from build123d import *

# Parameters (mm, degrees)
F1_DEPTH = 38.1


# Not quite as in the source:
# - the program builds the solid bodies; features that only make, move or delete a surface that nothing else refers to are left out


with BuildPart() as f1:
    # F0 (on Front) → F1 (new body)
    with BuildSketch(Plane.XZ):
        with BuildLine():
            Line((-12.4957701793, -2.2684196318), (12.4957701793, -2.2684196318))
            ThreePointArc((12.4957701793, -2.2684196318), (0, 12.7), (-12.4957701793, -2.2684196318))
        make_face()
        with BuildLine():
            Line((12.4957701793, -7.3484196318), (12.4957701793, -2.2684196318))
            Line((12.4957701793, -2.2684196318), (-12.4957701793, -2.2684196318))
            Line((-12.4957701793, -2.2684196318), (-49.8945600124, -2.2684196318))
            ThreePointArc((-49.8945600124, -2.2684196318), (-50.3994056233, -4.9895144213), (-51.8467453044, -7.3484196318))
            Line((-51.8467453044, -7.3484196318), (12.4957701793, -7.3484196318))
        make_face()
        with BuildLine():
            ThreePointArc((-51.8467453044, -7.3484196318), (-50.3994056233, -4.9895144213), (-49.8945600124, -2.2684196318))
            Line((-49.8945600124, -2.2684196318), (-57.4802711475, -2.2684196318))
            Line((-57.4802711475, -2.2684196318), (-57.4802711475, -7.3484196318))
            Line((-57.4802711475, -7.3484196318), (-51.8467453044, -7.3484196318))
        make_face()
        with BuildLine():
            Line((-57.4802711475, -2.2684196318), (-49.8945600124, -2.2684196318))
            ThreePointArc((-49.8945600124, -2.2684196318), (-64.5611366718, 0.4526751578), (-51.8467453044, -7.3484196318))
            Line((-51.8467453044, -7.3484196318), (-57.4802711475, -7.3484196318))
            Line((-57.4802711475, -7.3484196318), (-57.4802711475, -2.2684196318))
        make_face()
    extrude(amount=F1_DEPTH)


solid = f1.part
Work out the finished part from the listing and answer in its coordinate system (mm). A direction names the side the tool comes from. Coordinates: 2 decimals unless noted, no trailing zeros. Loops run counter-clockwise (first coordinate to the right, second up) from the corner with the lowest first, then second, coordinate; pieces in that order, holes last. Notation, with made-up numbers: (14, 44) -> (35, 44) arc R20 ccw to (35, 49) -> close; hole circle Ø3 at (36.25, 69). An arc over 180 degrees is marked (long way). Answer as CSV lines item,"result".
1) Straight lines are drawn through the part: probe 1 along Z at (x, y) = (-46, -11); probe 2 along X at (y, z) = (-21, -1.5); probe 3 along X at (y, z) = (-8.5, 2.75). For each, find the intervals that lie inside material, in ascending order.
A:
probe 1,"z = -7.35 to -2.27"
probe 2,"x = -65.03 to -49.93, -12.61 to 12.61"
probe 3,"x = -63.17 to -51.79, -12.4 to 12.4"
2) Flat-ended cylindrical pins translate along their axes: pin 1 (3 mm diameter, centred on x = -54, y = -19, fed in from -Z); pin 2 (11.5 mm diameter, centred on x = -35.5, y = -12, fed in from -Z); pin 3 (18.5 mm diameter, centred on x = -27, y = -19.5, fed in from +Z); pin 4 (12 mm diameter, centred on y = -7, z = 2, fed in from -X). Find the tip coordinate at first contact, or state that the pin passes through.
A:
pin 1,"stops at z = -9.59"
pin 2,"stops at z = -7.35"
pin 3,"stops at z = -2.27"
pin 4,"stops at x = -65.07"
3) The part is cut by section B-B (x = -41). Give the vertices of the cut face in (y, z).
A:
outline,"(-38.1, -7.35) -> (0, -7.35) -> (0, -2.27) -> (-38.1, -2.27) -> close"
4) For faces 1 (the face through (-20, -19, -7.348)), 2 (the face through (-64.45, -18.78, 0.73)), determine the directions among +Z, -Z, +X, -X, +Y, -Y from which every point of the face is accessible in a straight line to the end or side of a thin tool.
A:
face 1,"-Z, +X, +Y, -Y"
face 2,"+Y, -Y"
5) For a pull along X with two mould halves and no side action, classify faces 3 (the face through (12.496, -19, -5)), 4 (the face through (-18, -38.1, -3)), 5 (the face through (0.311, -18.783, 12.696)) as released by +X, released by -X, zero draft, split by the parting line, or undercut.
A:
face 3,"released by +X"
face 4,"zero draft"
face 5,"undercut"
6) The part is cut by section A-A (z = 3.75). Give the vertices of the cut face in (x, y).
A:
outline,"(-62.1, -38.1) -> (-52.86, -38.1) -> (-52.86, 0) -> (-62.1, 0) -> close; (-12.13, -38.1) -> (12.13, -38.1) -> (12.13, 0) -> (-12.13, 0) -> close"
7) The part is cut by section D-D (z = 0). Give the vertices of the cut face in (x, y).
A:
outline,"(-64.72, -38.1) -> (-50.24, -38.1) -> (-50.24, 0) -> (-64.72, 0) -> close; (-12.7, -38.1) -> (12.7, -38.1) -> (12.7, 0) -> (-12.7, 0) -> close"
8) The part is cut by section C-C (y = -34). Give the vertices of the cut face in (x, z), and give its area (4 significant figures).
A:
outline,"(-51.85, -7.35) -> (12.5, -7.35) -> (12.5, -2.27) arc R12.7 ccw (long way) to (-12.5, -2.27) -> (-49.89, -2.27) arc R7.59 ccw (long way) to start"
area,"811.5 mm²"
